from build123d import *

# Parameters (mm, degrees)
PAD_DEPTH            = 55
SKETCH015_R          = 1.75
POCKET002_DEPTH      = 7.001
POCKET002_DEPTH_BACK = 4.001
SKETCH016_R          = 3
POCKET003_DEPTH      = 4.5
CHAMFER002_SIZE      = 0.4


with BuildPart() as part:
    # Sketch014 → Pad (new body, symmetric)
    with BuildSketch(Plane.XZ):
        with BuildLine():
            ThreePointArc((-5.623508, -0.5), (-5.123508, 0), (-5.623508, 0.5))
            Line((-6.023508, 0.5), (-5.623508, 0.5))
            ThreePointArc((-6.023508, 0.5), (-6.223408, 0.992092), (-6.545786, 1.414214))
            Line((-7.5, 2.368427), (-6.545786, 1.414214))
            Line((-7.5, 3.5), (-7.5, 2.368427))
            Line((-7, 4), (-7.5, 3.5))
            Line((7, 4), (-7, 4))
            Line((7.5, 3.5), (7, 4))
            Line((7.5, 2.368427), (7.5, 3.5))
            Line((6.545786, 1.414214), (7.5, 2.368427))
            ThreePointArc((6.545786, 1.414214), (6.223408, 0.992092), (6.023508, 0.5))
            Line((5.623508, 0.5), (6.023508, 0.5))
            ThreePointArc((5.623508, 0.5), (5.123508, 0), (5.623508, -0.5))
            Line((5.623508, -0.5), (6.023508, -0.5))
            ThreePointArc((6.023508, -0.5), (6.560429, -1.428706), (7.5, -1.946381))
            Line((7.5, -6.5), (7.5, -1.946381))
            Line((7, -7), (7.5, -6.5))
            Line((-7, -7), (7, -7))
            Line((-7.5, -6.5), (-7, -7))
            Line((-7.5, -1.946381), (-7.5, -6.5))
            ThreePointArc((-7.5, -1.946381), (-6.560429, -1.428706), (-6.023508, -0.5))
            Line((-6.023508, -0.5), (-5.623508, -0.5))
        make_face()
    extrude(amount=PAD_DEPTH, both=True)

    # Sketch015 → Pocket002 (cut, two sides)
    with BuildSketch(Plane.XY) as pocket002_sk:
        with Locations((0, -40)):
            Circle(SKETCH015_R)
        Circle(SKETCH015_R)
        with Locations((0, 40)):
            Circle(SKETCH015_R)
    extrude(amount=-POCKET002_DEPTH, mode=Mode.SUBTRACT)
    extrude(pocket002_sk.sketch, amount=POCKET002_DEPTH_BACK, mode=Mode.SUBTRACT)

    # Sketch016 (on Face13 of Pocket002) → Pocket003 (cut)
    with BuildSketch(Plane(origin=(0, 0, 4), x_dir=(-1, 0, 0), z_dir=(0, 0, 1))):
        with Locations((0, 40)):
            Circle(SKETCH016_R)
        Circle(SKETCH016_R)
        with Locations((0, -40)):
            Circle(SKETCH016_R)
    extrude(amount=-POCKET003_DEPTH, mode=Mode.SUBTRACT)

    # Chamfer002
    chamfer002_edges = [part.edges().sort_by_distance(p)[0] for p in [
        (-1.75, -40, -7),
        (-1.75, 0, -7),
        (-1.75, 40, -7),
        (3, 40, 4),
        (3, 0, 4),
        (3, -40, 4),
    ]]
    chamfer(chamfer002_edges, length=CHAMFER002_SIZE)


solid = part.part
Part model, mm, in its own coordinate system. A direction names the side the tool comes from. Give positions to 0.01 mm unless a question says otherwise; leave off trailing zeros. Loops run counter-clockwise (first coordinate to the right, second up) from the corner with the lowest first, then second, coordinate; pieces in that order, holes last. Notation, with made-up numbers: M -36,45.5 L -21,45.5 A17 ccw -21,68.5 Z; hole C 54.5,57 d6. An arc over 180 degrees is marked long. Put each result on its own line as item: value. Start each with the question number.
1) Pull direction Y, two halves, no side cores. Call faces 3 (the cylindrical face through (-0.38, 38.29, -3.51)), 4 (the flat face through (0, -55, -1)), 5 (the flat face through (-7.5, -1, -4)): +Y half, -Y half, draft (parallel to the pull), parting line (faces both ways), or undercut.
2) Saw through at C-C (x = 0). State how many separate pieces and enclosed holes the cut face has, then the cut area to 3 significant figures.
3) Flat gauge pins, fed straight in: pin 1 (6.5 mm diameter, centred on x = 0, y = 1, fed in from +Z); pin 2 (4 mm diameter, centred on x = 0, y = -40, fed in from +Z). Where does each tip first touch, or does it go through?
4) 3-axis set-ups, long thin cutter, end or side, ignore diameter. For faces 1 (the flat face through (5, -1, 4)), 2 (the cylindrical face through (0, -43, 2)): which of +Z, -Z, +X, -X, +Y, -Y reach the whole face in a straight line?
5) Saw through at B-B (y = 15.5). List the corners of the cut face in (x, z), then the cut area to 3 significant figures.
6) Probe probe 1 along Y at (x, z) = (0, -4); probe 2 along Y at (x, z) = (0, 0.8); probe 3 along Z at (x, y) = (5.75, -32.5). List the from-to ranges inside material, lowest first.
Numbers:
1. face 3: undercut
1. face 4: -Y half
1. face 5: draft
2. separate pieces: 4
2. enclosed holes: 0
2. area: 1,060 mm^2
3. pin 1: z = 4
3. pin 2: z = -0.5
4. face 1: +Z, +X, -X, +Y, -Y
4. face 2: +Z
5. outline: M -7.5,-6.5 L -7,-7 L 7,-7 L 7.5,-6.5 L 7.5,-1.95 A2 cw 6.02,-0.5 L 5.62,-0.5 A0.5 cw 5.62,0.5 L 6.02,0.5 A2 cw 6.55,1.41 L 7.5,2.37 L 7.5,3.5 L 7,4 L -7,4 L -7.5,3.5 L -7.5,2.37 L -6.55,1.41 A2 cw -6.02,0.5 L -5.62,0.5 A0.5 cw -5.62,-0.5 L -6.02,-0.5 A2 cw -7.5,-1.95 Z
5. area: 154 mm^2
6. probe 1: -55 to -41.75, -38.25 to -1.75, 1.75 to 38.25, 41.75 to 55
6. probe 2: -55 to -43, -37 to -3, 3 to 37, 43 to 55
6. probe 3: -7 to -0.5, 0.5 to 4
